```python
from build123d import *

# Parameters (mm, degrees)
F1_DEPTH = 1.5875
F2_DEPTH = 2.38125
F0_R     = 4.8006
F3_DEPTH = 3.175


with BuildPart() as f1:
    # F0 (on Top) → F1 (new body, symmetric)
    with BuildSketch(Plane.XY):
        with BuildLine():
            Line((0, 110.85698), (0, 0))
            Line((0, 0), (-1.490273, -8.418053))
            ThreePointArc((-1.490273, -8.418053), (4.7625, -3.175), (11.015273, -8.418053))
            Line((11.015273, -8.418053), (9.525, 0))
            Line((9.525, 0), (9.525, 110.85698))
            Line((9.525, 110.85698), (12.762214, 121.829874))
            Line((12.762214, 121.829874), (13.417772, 124.051962))
            Line((13.417772, 124.051962), (14.2875, 127))
            ThreePointArc((14.2875, 127), (13.011392, 131.7625), (9.525, 135.248892))
            Line((9.525, 135.248892), (9.525, 124.051962))
            Line((9.525, 124.051962), (0, 124.051962))
            Line((0, 124.051962), (0, 135.248892))
            ThreePointArc((0, 135.248892), (-4.13073, 130.411172), (-4.294801, 124.051962))
            Line((-4.294801, 124.051962), (0, 110.85698))
        make_face()
    extrude(amount=F1_DEPTH, both=True)

    # F0 (on Top) → F2 (join, symmetric)
    with BuildSketch(Plane.XY):
        with BuildLine():
            Line((0, 110.85698), (0, 0))
            Line((0, 0), (-1.490273, -8.418053))
            ThreePointArc((-1.490273, -8.418053), (4.7625, -3.175), (11.015273, -8.418053))
            Line((11.015273, -8.418053), (9.525, 0))
            Line((9.525, 0), (9.525, 110.85698))
            Line((9.525, 110.85698), (12.762214, 121.829874))
            Line((12.762214, 121.829874), (13.417772, 124.051962))
            Line((13.417772, 124.051962), (14.2875, 127))
            ThreePointArc((14.2875, 127), (13.011392, 131.7625), (9.525, 135.248892))
            Line((9.525, 135.248892), (9.525, 124.051962))
            Line((9.525, 124.051962), (0, 124.051962))
            Line((0, 124.051962), (0, 135.248892))
            ThreePointArc((0, 135.248892), (-4.13073, 130.411172), (-4.294801, 124.051962))
            Line((-4.294801, 124.051962), (0, 110.85698))
        make_face()
    extrude(amount=F2_DEPTH, both=True)

    # F0 (on Top) → F3 (join, symmetric)
    with BuildSketch(Plane.XY):
        with BuildLine():
            ThreePointArc((11.015273, -8.418053), (4.7625, -3.175), (-1.490273, -8.418053))
            ThreePointArc((-1.490273, -8.418053), (4.206896, -15.850647), (11.1125, -9.525))
            ThreePointArc((11.1125, -9.525), (11.088147, -8.969396), (11.015273, -8.418053))
        make_face()
        with Locations((4.7625, -9.525)):
            Circle(F0_R, mode=Mode.SUBTRACT)
    extrude(amount=F3_DEPTH, both=True)


solid = f1.part
```
Check sheet for the modelled part. Datum: model origin and axes. Units: mm. A direction names the side the tool comes from. Round coordinates to 2 decimals unless told otherwise and drop trailing zeros. Order: outer loops, then holes, each group sorted by start corner. A loop starts at its lowest first (then second) coordinate and runs counter-clockwise, first axis right, second up. Notation, with made-up numbers: M 56.5,-39.5 L 92.5,-39.5 A19 cw 92.5,-5.5 Z; hole C 37.5,-20 d11. An arc over 180 degrees is marked long. Answer in a Markdown table with one row per item.
(1) Draft check along X on faces 1 (the flat face through (0, 56, 0)), 2 (the cylindrical face through (7.343, -5.477, -0.044)), 3 (the flat face through (5, 64, 2.381)). Enter one of: +X half, -X half, draft (parallel to the pull), parting line (faces both ways), or undercut.
Findings:
| item | result |
|---|---|
| face 1 | -X half |
| face 2 | undercut |
| face 3 | draft |
(2) Gauge pin test, flat ends, axial feed: pin 1 (1.4 mm diameter, centred on x = 4, z = 1, fed in from +Y); pin 2 (1 mm diameter, centred on x = -2, y = 2, fed in from +Z); pin 3 (1.5 mm diameter, centred on x = 3.5, z = -2, fed in from -Y); pin 4 (6 mm diameter, centred on x = 6, y = 46, fed in from +Z). Record the tip position at first contact, or that the pin passes through.
Findings:
| item | result |
|---|---|
| pin 1 | stops at y = 124.05 |
| pin 2 | passes through |
| pin 3 | stops at y = -15.85 |
| pin 4 | stops at z = 2.38 |
(3) Section check B-B on x = 7.5. Record the boundary of the cut face in (y, z) (3 decimals), plus the area to 3 significant figures.
Findings:
| item | result |
|---|---|
| outline | M -15.255,-3.175 L -13.469,-3.175 L -13.469,3.175 L -15.255,3.175 Z; M -5.581,-3.175 L -3.795,-3.175 L -3.795,-2.381 L 124.052,-2.381 L 124.052,2.381 L -3.795,2.381 L -3.795,3.175 L -5.581,3.175 Z |
| area | 632 mm^2 |
(4) Material ranges on line 1 along Z through (x, y) = (9.25, 42); line 2 along X through (y, z) = (49, -0.25) (3 decimals); line 3 along Y through (x, z) = (3.5, 2.5), recorded low to high. Write a range as from..to.
Findings:
| item | result |
|---|---|
| line 1 | z = -2.38..2.38 |
| line 2 | x = 0..9.525 |
| line 3 | y = -15.75..-14.16, -4.89..-3.3 |
(5) Section check D-D on y = 106.5. Record the boundary of the cut face in (x, z) (3 decimals), plus the area to 3 significant figures.
Findings:
| item | result |
|---|---|
| outline | M 0,-2.381 L 9.525,-2.381 L 9.525,2.381 L 0,2.381 Z |
| area | 45.4 mm^2 |
(6) Set-up check for faces 4 (the flat face through (10.28, -4.27, 0.03)), 5 (the flat face through (5, 124.052, 0)), 6 (the flat face through (2, -5, 3.175)), 7 (the flat face through (-2.18, 117.55, 0.03)), 8 (the flat face through (2, -5, -3.175)): record each of +Z, -Z, +X, -X, +Y, -Y from which the full face is reachable in a straight line by a thin tool's end or side.
Findings:
| item | result |
|---|---|
| face 4 | +Z, -Z, +X |
| face 5 | +Z, -Z, +Y |
| face 6 | +Z, +X, -X, +Y, -Y |
| face 7 | +Z, -Z, -X |
| face 8 | -Z, +X, -X, +Y, -Y |
(7) Section check C-C on y = -6. Record the boundary of the cut face in (x, z) (3 decimals).
Findings:
| item | result |
|---|---|
| outline | M -1.062,-2.381 L -0.519,-2.381 L -0.519,-3.175 L 1.504,-3.175 L 1.504,3.175 L -0.519,3.175 L -0.519,2.381 L -1.062,2.381 Z; M 8.021,-3.175 L 10.044,-3.175 L 10.044,-2.381 L 10.587,-2.381 L 10.587,2.381 L 10.044,2.381 L 10.044,3.175 L 8.021,3.175 Z |
